CAD build for the part. Positions are in the model's coordinates, mm. Face numbers are marked on the shaded views. A direction names the side the tool comes from. Give positions to 0.01 mm unless a question says otherwise; leave off trailing zeros. Loops run counter-clockwise (first coordinate to the right, second up) from the corner with the lowest first, then second, coordinate; pieces in that order, holes last. Notation, with made-up numbers: M -12.75,73 L 23.25,73 A23 cw 23.25,85 Z; hole C 73.5,21 d8. An arc over 180 degrees is marked long. Answer as CSV lines item,"result".
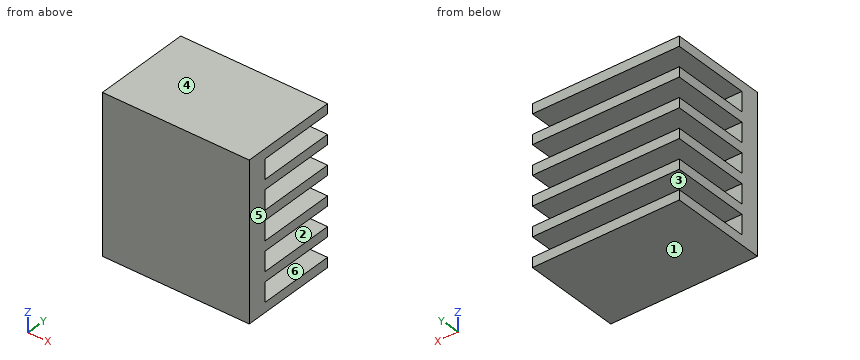
```python
from build123d import *

# Parameters (mm, degrees)
SKETCH1_W           = 75
SKETCH1_H           = 80
BOSS_EXTRUDE1_DEPTH = 50
SKETCH2_W           = 75
SKETCH2_H           = 10
CUT_EXTRUDE1_DEPTH  = 40


with BuildPart() as part:
    # Sketch1 → Boss-Extrude1 (new body)
    with BuildSketch(Plane(origin=(0, 0, 0), x_dir=(1, 0, 0), z_dir=(0, 1, 0))):
        Rectangle(SKETCH1_W, SKETCH1_H)
    extrude(amount=BOSS_EXTRUDE1_DEPTH)

    # Sketch2 → Cut-Extrude1 (cut)
    with BuildSketch(Plane(origin=(0, 50, 0), x_dir=(1, 0, 0), z_dir=(0, 1, 0))):
        with Locations((0, 30)):
            Rectangle(SKETCH2_W, SKETCH2_H)
        with Locations((0, 15)):
            Rectangle(SKETCH2_W, SKETCH2_H)
        Rectangle(SKETCH2_W, SKETCH2_H)
        with Locations((0, -15)):
            Rectangle(SKETCH2_W, SKETCH2_H)
        with Locations((0, -30)):
            Rectangle(SKETCH2_W, SKETCH2_H)
    extrude(amount=-CUT_EXTRUDE1_DEPTH, mode=Mode.SUBTRACT)


solid = part.part
```
Q1. Cut at A-A (y = 13). Write the cut outline in (x, z).
Solution:
outline,"M -37.5,-40 L 37.5,-40 L 37.5,-35 L -37.5,-35 Z; M -37.5,-25 L 37.5,-25 L 37.5,-20 L -37.5,-20 Z; M -37.5,-10 L 37.5,-10 L 37.5,-5 L -37.5,-5 Z; M -37.5,5 L 37.5,5 L 37.5,10 L -37.5,10 Z; M -37.5,20 L 37.5,20 L 37.5,25 L -37.5,25 Z; M -37.5,35 L 37.5,35 L 37.5,40 L -37.5,40 Z"
Q2. Pin check, flat tip, straight feed: P1, Ø3, axis at x = -9.5, z = -15.5, coming from the +Y side. Stop position of the tip, or through.
Solution:
P1,"stops at y = 10"
Q3. Mould opens along Z. For the marked faces 3, 4, 5 and 6 say: released by +Z, released by -Z, zero draft, split by the parting line, or undercut.
Solution:
face 3,"undercut"
face 4,"released by +Z"
face 5,"zero draft"
face 6,"undercut"
Q4. Cut at C-C (z = 15). Write the cut outline in (x, y), and give its area (3 significant figures).
Solution:
outline,"M -37.5,0 L 37.5,0 L 37.5,10 L -37.5,10 Z"
area,"750 mm²"
Q5. Which spindle directions (+Z, -Z, +X, -X, +Y, -Y) get a long thin tool onto all of the face, cutting with end or side? Do the marked faces 1 and 2. Say none if no direction does.
Solution:
face 1,"-Z, +X, -X, +Y, -Y"
face 2,"+X, -X, +Y"
Q6. Wall check: line 1 (Z direction, x = -27, y = 11); line 2 (Y direction, x = 25.5, z = 2). Give the ranges that are in metal, low to high. Write a range as [from, to].
Solution:
line 1,"z = [-40, -35], [-25, -20], [-10, -5], [5, 10], [20, 25], [35, 40]"
line 2,"y = [0, 10]"
Q7. Cut at B-B (x = -1.5). Write the cut outline in (y, z), and give its area (3 significant figures).
Solution:
outline,"M 0,-40 L 50,-40 L 50,-35 L 10,-35 L 10,-25 L 50,-25 L 50,-20 L 10,-20 L 10,-10 L 50,-10 L 50,-5 L 10,-5 L 10,5 L 50,5 L 50,10 L 10,10 L 10,20 L 50,20 L 50,25 L 10,25 L 10,35 L 50,35 L 50,40 L 0,40 Z"
area,"2,000 mm²"
